Source: CAD feature listing. Evaluate the final solid. Frame: model axes, mm. A direction names the side the tool comes from. Coordinates: 2 decimals unless noted, no trailing zeros. Loops run counter-clockwise (first coordinate to the right, second up) from the corner with the lowest first, then second, coordinate; pieces in that order, holes last.
Item 1: Line query: probe 1 along Y at (x, z) = (0, 0.9); probe 2 along X at (y, z) = (3, 1.05); probe 3 along X at (y, z) = (4, 1.1). Output: solid intervals per line, ascending.
Item 2: Section query B-B, the plane y = 12.25. Return the cut outline in (x, z), then the cut area to 3 significant figures.
Item 3: Section query D-D, the plane x = -9. Return the cut outline in (y, z).
Item 4: Pull-direction query (X, two-part tool) for faces 1 (the cylindrical face through (-34.388, 10.665, 0.789)), 2 (the flat face through (26.84, 8.88, 3)), 3 (the flat face through (0, 6.205, 1)); classes: +X half, -X half, draft (parallel to the pull), parting line (faces both ways), or undercut.
Item 5: Section query C-C, the plane z = 0.8. Return the cut outline in (x, y), then the cut area to 3 significant figures.
Item 6: Pin query (flat end, axial travel): pin 1 Ø8.5 at (x, y) = (0, 0) entering from +Z; pin 2 Ø2.5 at (x, y) = (8.41, 3.48) entering from +Z; pin 3 Ø1 at (x, z) = (-27.5, 1.5) entering from -Y; pin 4 Ø0.5 at (x, z) = (-0.5, 0.5) entering from +Y. Return the tip coordinate at first contact, or that it passes through.
Item 7: Section query A-A, the plane x = 0. Return the cut outline in (y, z).
Item 8: Reachability of faces 4 (the flat face through (-29.17, 16.86, 0.79)), 5 (the cylindrical face through (-23.7, 9.81, 2.29)), 6 (the flat face through (6.413, -4.657, 0.789)), 7 (the flat face through (-6.43, -4.7, 0.79)) from +Z, -Z, +X, -X, +Y, -Y: full face, straight path, thin tool, end or side. Return the list, or none.
```python
from build123d import *

# Parameters (mm, degrees)
SKETCH1_R             = 2.6
BOSS_EXTRUDE1_DEPTH   = 1.6
SKETCH2_R             = 3.45
BOSS_EXTRUDE2_DEPTH   = 1.4
M5X0_8_TAPPED_HOLE1_D = 4.2


with BuildPart() as part:
    # Sketch1 → Boss-Extrude1 (new body)
    with BuildSketch(Plane.XY):
        with BuildLine():
            Line((-1.9135, 6.204558653), (1.9135, 6.204558653))
            Line((1.9135, 6.204558653), (27.320187144, 16.728353043))
            Line((27.320187144, 16.728353043), (30.973251278, 16.987968318))
            ThreePointArc((30.973251278, 16.987968318), (31.868181477, 16.767718217), (32.465404107, 16.065767153))
            Line((32.465404107, 16.065767153), (34.316720297, 11.596294499))
            ThreePointArc((34.316720297, 11.596294499), (34.390774483, 10.67763997), (33.91370361, 9.889088418))
            Line((33.91370361, 9.889088418), (31.147021468, 7.489557718))
            Line((31.147021468, 7.489557718), (5.740334324, -3.034236672))
            Line((5.740334324, -3.034236672), (7.103934305, -6.32625824))
            ThreePointArc((7.103934305, -6.32625824), (7.015220781, -7.226981758), (6.217009953, -7.653634335))
            Line((6.217009953, -7.653634335), (-6.217009953, -7.653634335))
            ThreePointArc((-6.217009953, -7.653634335), (-7.015220781, -7.226981758), (-7.103934305, -6.32625824))
            Line((-7.103934305, -6.32625824), (-5.740334324, -3.034236672))
            Line((-5.740334324, -3.034236672), (-31.147021468, 7.489557718))
            Line((-31.147021468, 7.489557718), (-33.91370361, 9.889088418))
            ThreePointArc((-33.91370361, 9.889088418), (-34.390774483, 10.67763997), (-34.316720297, 11.596294499))
            Line((-34.316720297, 11.596294499), (-32.465404107, 16.065767153))
            ThreePointArc((-32.465404107, 16.065767153), (-31.868181477, 16.767718217), (-30.973251278, 16.987968318))
            Line((-30.973251278, 16.987968318), (-27.320187144, 16.728353043))
            Line((-27.320187144, 16.728353043), (-1.9135, 6.204558653))
        make_face()
        Circle(SKETCH1_R, mode=Mode.SUBTRACT)
    extrude(amount=BOSS_EXTRUDE1_DEPTH)

    # Sketch2 → Boss-Extrude2 (add)
    with BuildSketch(Plane.XY.offset(1.6)):
        with Locations((26.884894396, 11.136087882)):
            Circle(SKETCH2_R)
        with Locations((8.407303746, 3.482419235)):
            Circle(SKETCH2_R)
        with Locations((-8.407303746, 3.482419235)):
            Circle(SKETCH2_R)
        with Locations((-26.884894396, 11.136087882)):
            Circle(SKETCH2_R)
    extrude(amount=BOSS_EXTRUDE2_DEPTH)

    # M5x0.8 Tapped Hole1 (through all)
    with Locations(Plane.XY.offset(3)):
        with Locations((26.884894396, 11.136087882), (8.407303746, 3.482419235), (-8.407303746, 3.482419235), (-26.884894396, 11.136087882)):
            Hole(M5X0_8_TAPPED_HOLE1_D / 2)


solid = part.part
```
Verdict:
1. probe 1: y = -7.65 to -2.6, 2.6 to 6.2
1. probe 2: x = -20.31 to -10.45, -6.36 to 6.36, 10.45 to 20.31
1. probe 3: x = -22.72 to -10.44, -6.37 to 6.37, 10.44 to 22.72
2. outline: (-34.05, 0) - (-28.67, 0) - (-28.67, 3) - (-30.15, 3) - (-30.15, 1.6) - (-34.05, 1.6) - close; (-25.1, 0) - (-16.51, 0) - (-16.51, 1.6) - (-23.62, 1.6) - (-23.62, 3) - (-25.1, 3) - close; (16.51, 0) - (25.1, 0) - (25.1, 3) - (23.62, 3) - (23.62, 1.6) - (16.51, 1.6) - close; (28.67, 0) - (34.05, 0) - (34.05, 1.6) - (30.15, 1.6) - (30.15, 3) - (28.67, 3) - close
2. area: 53.0 mm2
3. outline: (-1.68, 0) - (1.47, 0) - (1.47, 3) - (0.08, 3) - (0.08, 1.6) - (-1.68, 1.6) - close; (5.5, 0) - (9.14, 0) - (9.14, 1.6) - (6.88, 1.6) - (6.88, 3) - (5.5, 3) - close
4. face 1: -X half
4. face 2: draft
4. face 3: undercut
5. outline: (-34.32, 11.6) arc R1.5 ccw to (-33.91, 9.89) - (-31.15, 7.49) - (-5.74, -3.03) - (-7.1, -6.33) arc R0.96 ccw to (-6.22, -7.65) - (6.22, -7.65) arc R0.96 ccw to (7.1, -6.33) - (5.74, -3.03) - (31.15, 7.49) - (33.91, 9.89) arc R1.5 ccw to (34.32, 11.6) - (32.47, 16.07) arc R1.5 ccw to (30.97, 16.99) - (27.32, 16.73) - (1.91, 6.2) - (-1.91, 6.2) - (-27.32, 16.73) - (-30.97, 16.99) arc R1.5 ccw to (-32.47, 16.07) - close; hole circle Ø4.2 at (-26.88, 11.14); hole circle Ø4.2 at (-8.41, 3.48); hole circle Ø5.2 at (0, 0); hole circle Ø4.2 at (8.41, 3.48); hole circle Ø4.2 at (26.88, 11.14)
5. area: 681 mm2
6. pin 1: stops at z = 1.6
6. pin 2: passes through
6. pin 3: stops at y = 5.77
6. pin 4: stops at y = 6.2
7. outline: (-7.65, 0) - (-2.6, 0) - (-2.6, 1.6) - (-7.65, 1.6) - close; (2.6, 0) - (6.2, 0) - (6.2, 1.6) - (2.6, 1.6) - close
8. face 4: +Z, -Z, +Y
8. face 5: +Z
8. face 6: +Z, -Z, +X
8. face 7: +Z, -Z, -X
